Here's how the part is built. I have some questions about the finished solid (model axes, mm). A direction names the side the tool comes from. Give positions to 0.01 mm unless a question says otherwise; leave off trailing zeros. Order: outer loops, then holes, each group sorted by start corner. A loop starts at its lowest first (then second) coordinate and runs counter-clockwise, first axis right, second up. Notation, with made-up numbers: (-33, 17) - (22, 17) arc R27 ccw to (22, 34) - close; hole circle Ø6 at (76, 17.5). An arc over 180 degrees is marked (long way). One line per question, with ' | ' between items.
from build123d import *

# Parameters (mm, degrees)
SKETCH1_R           = 15.875
BOSS_EXTRUDE1_DEPTH = 20.32
SKETCH2_W           = 15.252884162
SKETCH2_H           = 18.365256134
BOSS_EXTRUDE2_DEPTH = 2.54


with BuildPart() as part:
    # Sketch1 → Boss-Extrude1 (new body)
    with BuildSketch(Plane(origin=(0, 0, 0), x_dir=(1, 0, 0), z_dir=(0, 1, 0))):
        with Locations(Location((0, 0, 0), (0, 0, 270))):
            Circle(SKETCH1_R)
    extrude(amount=BOSS_EXTRUDE1_DEPTH)

    # Sketch2 → Boss-Extrude2 (add)
    with BuildSketch(Plane.XZ):
        with Locations((15.875, 0)):
            Rectangle(SKETCH2_W, SKETCH2_H)
    extrude(amount=-BOSS_EXTRUDE2_DEPTH)


solid = part.part
1) I want a section at B-B (z = 0). List the corners of the cut face in (x, y) for me (3 decimals), plus the area to 3 significant figures.
Model answer:
outline: (-15.875, 0) - (23.501, 0) - (23.501, 2.54) - (15.875, 2.54) - (15.875, 20.32) - (-15.875, 20.32) - close | area: 665 mm2
2) I want a section at D-D (z = 4). List the corners of the cut face in (x, y) for me, plus the area to 3 significant figures.
Model answer:
outline: (-15.36, 0) - (23.5, 0) - (23.5, 2.54) - (15.36, 2.54) - (15.36, 20.32) - (-15.36, 20.32) - close | area: 645 mm2
3) On a 3-axis mill with a long thin cutter (end or side, diameter ignored), from which of +Z, -Z, +X, -X, +Y, -Y can I reach the whole of each face in a straight line? I mean faces 1 (the face through (18, 1, -9.183)), 2 (the face through (18, 1, 9.183)), 3 (the face through (4, 0, 0)), 4 (the face through (-15.497, 10.018, -3.441)). Say none if no direction works.
Model answer:
face 1: -Z, +X, +Y, -Y | face 2: +Z, +X, +Y, -Y | face 3: +Z, -Z, +X, -X, -Y | face 4: +Y
4) I want a section at C-C (x = 11.5). List the corners of the cut face in (y, z) for me, plus the area to 3 significant figures.
Model answer:
outline: (0, -10.94) - (20.32, -10.94) - (20.32, 10.94) - (0, 10.94) - close | area: 445 mm2
5) I want a section at A-A (y = 6). List the corners of the cut face in (x, z) for me (3 decimals).
Model answer:
outline: circle Ø31.75 at (0, 0)
6) Please list where these lines run through material, in increasing order: L1, parallel to Y at x = 21.5, z = -8.5; L2, parallel to X at y = 3, z = -8; L3, parallel to X at y = 16, z = 3.
Model answer:
L1: y = 0 to 2.54 | L2: x = -13.71 to 13.71 | L3: x = -15.59 to 15.59
7) I'm going to push flat-ended pins straight in: P1, Ø3, axis at x = 18, y = 2, coming from the +Z side; P2, Ø5.5, axis at x = 18.5, z = 3.5, coming from the +Y side; P3, Ø3, axis at y = 18, z = -4, coming from the +X side. Where does each tip first touch, or does it pass through?
Model answer:
P1: stops at z = 9.18 | P2: stops at y = 2.54 | P3: stops at x = 15.68
